from build123d import *

# Parameters (mm, degrees)
F1_DEPTH  = 42.3
F3_W      = 30.3
F3_H      = 6
F4_DEPTH  = 6
F2_W      = 30.3
F2_H      = 6
F5_DEPTH  = 12
F6_SIZE   = 5.99999
F7_R      = 1.5
F8_DEPTH  = 8.501
F9_R      = 1.5
F10_DEPTH = 8.501
F11_R     = 1.5
F11_R_2   = 7.5
F12_DEPTH = 5
F13_SIZE  = 5


# Not quite as in the source:
# - a fillet or chamfer is up to 0.001 mm smaller than in the source, because OpenCascade refuses the exact size
# - a feature names something its author has since deleted; it is built from what else it names


with BuildPart() as f1:
    # F0 (on Right) → F1 (new body)
    with BuildSketch(Plane.YZ):
        Polygon((-9.5, 9.5), (0, 9.5), (0, 14.5), (-14.5, 14.5), (-20.5, 14.5), (-20.5, 8.5), (-62.8, 8.5), (-62.8, 3.5), (-20.5, 3.5), (-20.5, -2.5), (-14.5, -2.5), (-14.5, -14.5), (0, -14.5), (0, -9.5), (-9.5, -9.5), align=None)
    extrude(amount=F1_DEPTH)

    # F3 (on face) → F4 (cut)
    with BuildSketch(Plane.XZ.offset(14.5)):
        with Locations((21.15, -11.5)):
            Rectangle(F3_W, F3_H)
    extrude(amount=-F4_DEPTH, mode=Mode.SUBTRACT)

    # F2 (on face) → F5 (cut)
    with BuildSketch(Plane.XZ.offset(20.5)):
        with Locations((21.15, 11.5)):
            Rectangle(F2_W, F2_H)
    extrude(amount=-F5_DEPTH, mode=Mode.SUBTRACT)

    # F6 (size 6 in the source; OpenCascade refuses exactly that, so slightly less here)
    f6_edges = [f1.edges().sort_by_distance(p)[0] for p in [
        (3, -14.5, -14.5),
        (39.3, -14.5, -14.5),
        (3, -20.5, 14.5),
        (39.3, -20.5, 14.5),
        (21.15, -20.5, -2.5),
    ]]
    chamfer(f6_edges, length=F6_SIZE)

    # F7 (on face) → F8 (cut, through all)
    with BuildSketch(Plane.XZ.offset(8.5)):
        with Locations((10.5, 12)):
            Circle(F7_R)
        with Locations((31.8, 12)):
            Circle(F7_R)
    extrude(amount=-F8_DEPTH, mode=Mode.SUBTRACT)

    # F9 (on face) → F10 (cut, through all)
    with BuildSketch(Plane.XZ.offset(8.5)):
        with Locations((10.5, -12)):
            Circle(F9_R)
        with Locations((31.8, -12)):
            Circle(F9_R)
    extrude(amount=-F10_DEPTH, mode=Mode.SUBTRACT)

    # F11 (on face) → F12 (cut, through all)
    with BuildSketch(Plane.XY.offset(8.5)):
        with Locations((8.1596189432, -34.15)):
            Circle(F11_R)
        with Locations((21.15, -41.65)):
            Circle(F11_R_2)
        with Locations((34.1403810568, -34.15)):
            Circle(F11_R)
        with Locations((21.15, -56.65)):
            Circle(F11_R)
    extrude(amount=-F12_DEPTH, mode=Mode.SUBTRACT)

    # F13
    f13_edges = [f1.edges().sort_by_distance(p)[0] for p in [
        (42.3, -62.8, 6),
        (0, -62.8, 6),
    ]]
    chamfer(f13_edges, length=F13_SIZE)


solid = f1.part
Can you work these out from the model? Positions are in its coordinate system, mm. A direction names the side the tool comes from. Give positions to 0.01 mm unless a question says otherwise; leave off trailing zeros. Loops run counter-clockwise (first coordinate to the right, second up) from the corner with the lowest first, then second, coordinate; pieces in that order, holes last. Notation, with made-up numbers: (-36, -22.5) - (-8, -22.5) arc R29 cw to (-8, 4.5) - close; hole circle Ø9 at (82.5, 69.25). An arc over 180 degrees is marked (long way). Return JSON: item names as keys, results as strings.
1. I want a section at D-D on y = -4.5. Please give me the cut outline in (x, z), and give its area (3 significant figures).
Output values:
{"outline": "(0, -14.5) - (42.3, -14.5) - (42.3, -9.5) - (0, -9.5) - close; (0, 9.5) - (42.3, 9.5) - (42.3, 14.5) - (0, 14.5) - close; hole circle Ø3 at (10.5, -12); hole circle Ø3 at (10.5, 12); hole circle Ø3 at (31.8, -12); hole circle Ø3 at (31.8, 12)", "area": "395 mm²"}
2. I want a section at C-C on z = -12. Please give me the cut outline in (x, y).
Output values:
{"outline": "(0, -11) - (6, -11) - (6, -8.5) - (9, -8.5) - (9, 0) - (0, 0) - close; (12, -8.5) - (30.3, -8.5) - (30.3, 0) - (12, 0) - close; (33.3, -8.5) - (36.3, -8.5) - (36.3, -11) - (42.3, -11) - (42.3, 0) - (33.3, 0) - close"}
3. We'd pull the mould along Z, two halves only. Please class faces 1 (the face through (9, -4, 12)), 2 (the face through (9.59, -33.7, 6.04)), 3 (the face through (21, -12, -8.5)): +Z half, -Z half, draft (parallel to the pull), parting line (faces both ways), or undercut.
Output values:
{"face 1": "undercut", "face 2": "draft", "face 3": "-Z half"}
4. I want a section at B-B on x = 21.15. Give the number of separate pieces and of enclosed holes in the cut face, and give its area (4 significant figures).
Output values:
{"separate pieces": "5", "enclosed holes": "0", "area": "339.5 mm²"}
5. I want a section at A-A on y = -41.65. Please give me the cut outline in (x, z), and give its area (4 significant figures).
Output values:
{"outline": "(0, 3.5) - (13.65, 3.5) - (13.65, 8.5) - (0, 8.5) - close; (28.65, 3.5) - (42.3, 3.5) - (42.3, 8.5) - (28.65, 8.5) - close", "area": "136.5 mm²"}
6. For faces 4 (the face through (21, -14.5, -5)), 5 (the face through (6, -13, 11)), 6 (the face through (36.3, -10, -10)), which set-ups out of +Z, -Z, +X, -X, +Y, -Y let a thin tool reach every point of the face, with its end or its side?
Output values:
{"face 4": "-Z, +X, -X, -Y", "face 5": "+Z, -Y", "face 6": "-Z, -Y"}
7. I'm going to push flat-ended pins straight in: pin 1 Ø3 at (x, z) = (10, 11) entering from -Y; pin 2 Ø5 at (x, y) = (18, -56) entering from -Z; pin 3 Ø1.5 at (x, z) = (35.5, 4.5) entering from +Y. Where does each tip first touch, or does it pass through?
Output values:
{"pin 1": "stops at y = -8.5", "pin 2": "stops at z = 3.5", "pin 3": "stops at y = -9.5"}
8. If I drill on line 1 (Y direction, x = 21.15, z = 6.35); line 2 (Z direction, x = 10.5, y = -5.25); line 3 (Z direction, x = 31, y = -4), over which ranges is the centre line in solid material (lowest first)?
Output values:
{"line 1": "y = -62.8 to -58.15, -55.15 to -49.15, -34.15 to -9.5", "line 2": "z = -14.5 to -13.5, -10.5 to -9.5, 9.5 to 10.5, 13.5 to 14.5", "line 3": "z = -14.5 to -13.27, -10.73 to -9.5, 9.5 to 10.73, 13.27 to 14.5"}
